Verification items for the finished model (mm, model axes). Give positions to 0.01 mm unless a question says otherwise; leave off trailing zeros. Write each loop counter-clockwise with the first axis right and the second up, starting at its lowest first coordinate (ties: lowest second). Pieces come first, ordered by that corner, then holes. Notation, with made-up numbers: M -20.5,37.5 L 14.5,37.5 A22 ccw 14.5,62.5 Z; hole C -39,58.5 d3. An arc over 180 degrees is marked long. Write item = value, one per line.
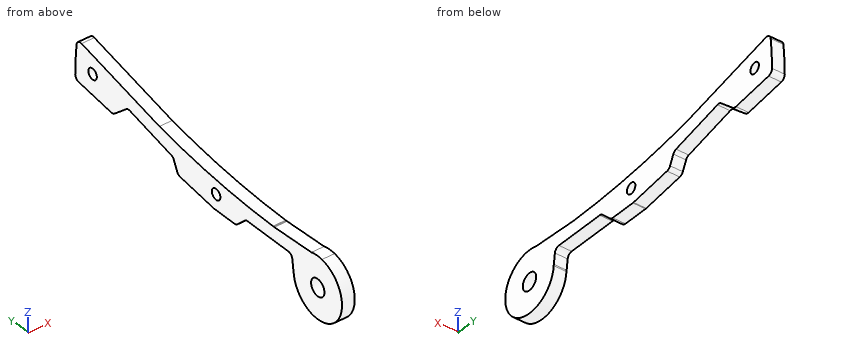
from build123d import *

# Parameters (mm, degrees)
F0_R     = 3.3
F0_R_2   = 2.1
F1_DEPTH = 5


# Not quite as in the source:
# - a feature names something its author has since deleted; it is built from what else it names


with BuildPart() as f1:
    # F0 (on Right) → F1 (new body)
    with BuildSketch(Plane.YZ):
        with BuildLine():
            ThreePointArc((21.8315579223, 10.717182122), (21.897134346, 10.7177196915), (21.9626931438, 10.7193322557))
            ThreePointArc((21.9626931438, 10.7193322557), (21.9630378123, 10.7252568669), (21.9633808826, 10.731181571))
            ThreePointArc((21.9633808826, 10.731181571), (21.7716697335, 10.7299327404), (21.5799577929, 10.728811993))
            Line((21.5799577929, 10.728811993), (21.8315579223, 10.717182122))
        make_face()
        with BuildLine():
            ThreePointArc((22.1844688263, 10.7327808001), (22.0736743793, 10.7245163933), (21.9626931438, 10.7193322557))
            ThreePointArc((21.9626931438, 10.7193322557), (21.897134346, 10.7177196915), (21.8315579223, 10.717182122))
            ThreePointArc((21.8315579223, 10.717182122), (21.6468606164, 10.7214485341), (21.4625573078, 10.7342386694))
            Line((21.4625573078, 10.7342386694), (3.1432257368, 11.581024651))
            Line((3.1432257368, 11.581024651), (-2.0614712889, 11.8216046341))
            ThreePointArc((-2.0614712889, 11.8216046341), (-7.9885695505, -8.9544824829), (11.9792964571, -0.7045966171))
            ThreePointArc((11.9792964571, -0.7045966171), (12.0074816864, -0.4822378377), (12.0652655082, -0.2656763826))
            Line((12.0652655082, -0.2656763826), (12.5823545671, 3.7402298466))
            ThreePointArc((12.5823545671, 3.7402298466), (13.2453067327, 4.9862024463), (14.565897859, 5.4841907695))
            Line((14.565897859, 5.4841907695), (34.746018001, 5.4841907695))
            ThreePointArc((34.746018001, 5.4841907695), (35.4911723527, 5.3401931919), (36.1290262829, 4.9289357615))
            Line((36.1290262829, 4.9289357615), (39.7961525429, 1.4185128035))
            ThreePointArc((39.7961525429, 1.4185128035), (40.4340064731, 1.0072553731), (41.1791608249, 0.8632577956))
            Line((41.1791608249, 0.8632577956), (51.1560065331, 0.8632577956))
            ThreePointArc((51.1560065331, 0.8632577956), (51.3046360431, 0.8687881245), (51.452443583, 0.8853485268))
            Line((51.452443583, 0.8853485268), (68.043755982, 3.3719538424))
            ThreePointArc((68.043755982, 3.3719538424), (68.9480745213, 3.750430082), (69.5639006382, 4.5131846154))
            Line((69.5639006382, 4.5131846154), (71.1927053136, 8.0496168184))
            ThreePointArc((71.1927053136, 8.0496168184), (71.7304115705, 8.7506241115), (72.5176709464, 9.151575379))
            Line((72.5176709464, 9.151575379), (93.0016589096, 14.3460792675))
            ThreePointArc((93.0016589096, 14.3460792675), (93.9531599103, 14.3538506609), (94.800564285, 13.9210454222))
            Line((94.800564285, 13.9210454222), (100.5567479715, 8.9494668086))
            ThreePointArc((100.5567479715, 8.9494668086), (101.3078443235, 8.5419637232), (102.1604743235, 8.4851607509))
            Line((102.1604743235, 8.4851607509), (118.2931486533, 10.9030281733))
            ThreePointArc((118.2931486533, 10.9030281733), (119.516973098, 11.5813971433), (119.9966558679, 12.8958685851))
            ThreePointArc((119.9966558679, 12.8958685851), (119.8113324935, 18.7264110882), (119.3428752162, 24.5410579746))
            ThreePointArc((119.3428752162, 24.5410579746), (118.5020303548, 25.9696085801), (116.872434029, 26.2732411356))
            Line((116.872434029, 26.2732411356), (78.344444671, 16.7187866332))
            ThreePointArc((78.344444671, 16.7187866332), (50.4120849121, 12.3407543123), (22.1844688263, 10.7327808001))
        make_face()
        Circle(F0_R, mode=Mode.SUBTRACT)
        with Locations((50.3031872213, 6.8563437089)):
            Circle(F0_R_2, mode=Mode.SUBTRACT)
        with Locations((111.4225909114, 17.8264938295)):
            Circle(F0_R_2, mode=Mode.SUBTRACT)
        with BuildLine():
            ThreePointArc((21.9633808826, 10.731181571), (21.9630378123, 10.7252568669), (21.9626931438, 10.7193322557))
            ThreePointArc((21.9626931438, 10.7193322557), (22.0736743793, 10.7245163933), (22.1844688263, 10.7327808001))
            ThreePointArc((22.1844688263, 10.7327808001), (22.0739250085, 10.7319598925), (21.9633808826, 10.731181571))
        make_face()
        with BuildLine():
            ThreePointArc((21.4625573078, 10.7342386694), (21.6468606164, 10.7214485341), (21.8315579223, 10.717182122))
            Line((21.8315579223, 10.717182122), (21.5799577929, 10.728811993))
            Line((21.5799577929, 10.728811993), (21.4625573078, 10.7342386694))
        make_face()
        with BuildLine():
            Line((-2.0614712889, 11.8216046341), (3.1432257368, 11.581024651))
            ThreePointArc((3.1432257368, 11.581024651), (0.5540919179, 11.9872007636), (-2.0614712889, 11.8216046341))
        make_face()
    extrude(amount=F1_DEPTH)


solid = f1.part
1) Cross-section at A-A on y = 0. Record the boundary of the cut face in (x, z).
From the geometry:
outline = M 0,-12 L 5,-12 L 5,-3.3 L 0,-3.3 Z; M 0,3.3 L 5,3.3 L 5,12 L 0,12 Z
2) Depth check by flat-ended pin: P1, Ø4, axis at y = 72, z = 4, coming from the +X side; P2, Ø6.5, axis at y = 50.3, z = 6.86, coming from the +X side; P3, Ø2.5, axis at x = 3.5, y = 28, coming from the -Z side; P4, Ø2, axis at x = 4, y = 61.5, coming from the -Z side. Enter the tip coordinate at first touch or a pass-through.
From the geometry:
P1 = through
P2 = 5
P3 = 5.48
P4 = 2.24
3) Cross-section at C-C on y = 91. Record the boundary of the cut face in (x, z).
From the geometry:
outline = M 0,13.84 L 5,13.84 L 5,19.86 L 0,19.86 Z
4) Cross-section at B-B on x = 2.6. Count the separate pieces of the cut face and the enclosed holes in it, plus the area to 3 significant figures.
From the geometry:
separate_pieces = 1
enclosed_holes = 3
area = 1,420 mm^2
5) Cross-section at D-D on y = 75.5. Record the boundary of the cut face in (x, z), plus the area to 3 significant figures.
From the geometry:
outline = M 0,9.91 L 5,9.91 L 5,16.14 L 0,16.14 Z
area = 31.2 mm^2
6) Material ranges on probe 1 along Z at (x, y) = (1.8, 0); probe 2 along Y at (x, z) = (3.1, 6.5); probe 3 along Z at (x, y) = (2.35, 30), recorded low to high. Write a range as from..to.
From the geometry:
probe_1 = -12..-3.3, 3.3..12
probe_2 = -10.09..48.23, 52.37..70.48
probe_3 = 5.48..10.9
